from build123d import *

# Parameters (mm, degrees)
F0_R     = 11.6
F0_R_2   = 9.6
F1_DEPTH = 5.2
F2_R     = 11.6
F2_R_2   = 9.6
F3_DEPTH = 2
F4_W     = 40
F4_H     = 25
F4_R     = 11.6
F5_DEPTH = 7.2
F7_DEPTH = 1
F9_DEPTH = 1


with BuildPart() as f1:
    # F0 (on Top) → F1 (new body)
    with BuildSketch(Plane.XY):
        Circle(F0_R)
        Circle(F0_R_2, mode=Mode.SUBTRACT)
    extrude(amount=F1_DEPTH)

    # F2 (on face) → F3 (join)
    with BuildSketch(Plane.XY.offset(5.2)):
        Circle(F2_R)
        Circle(F2_R_2, mode=Mode.SUBTRACT)
        Circle(F2_R_2)
    extrude(amount=F3_DEPTH)

    # F4 (on face) → F5 (join)
    with BuildSketch(Plane.XY.offset(7.2)):
        Rectangle(F4_W, F4_H)
        Circle(F4_R, mode=Mode.SUBTRACT)
    extrude(amount=-F5_DEPTH)

    # F6 (on face) → F7 (cut)
    with BuildSketch(Plane.XY.offset(7.2)):
        Polygon((0, 2.9988845345), (-20, -12.5), (20, -12.5), align=None)
    extrude(amount=-F7_DEPTH, mode=Mode.SUBTRACT)

    # F8 (on face) → F9 (join)
    with BuildSketch(Plane.XY.offset(7.2)):
        Polygon((20, 12.5), (-20, 12.5), (-4.2277933686, -0.2774195283), (0, 2.9988845345), (4.2277933686, -0.2774195283), align=None)
        Polygon((0, 2.9988845345), (-4.2277933686, -0.2774195283), (0, -3.702450078), (4.2277933686, -0.2774195283), align=None)
    extrude(amount=F9_DEPTH)


solid = f1.part
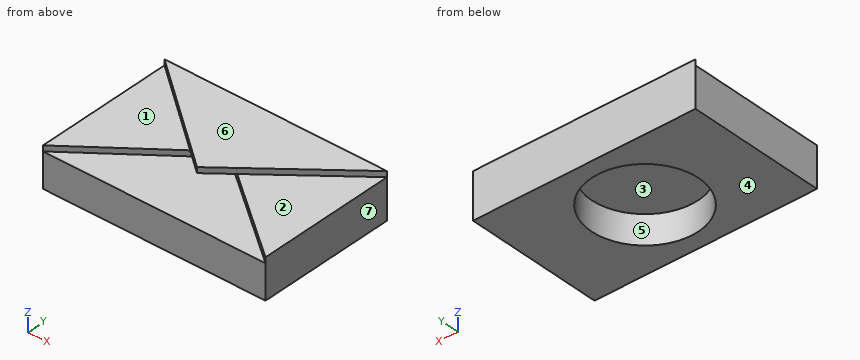
The model under review builds one solid part; all positions refer to its coordinate system, in mm. Face numbers are marked on the shaded views. A direction names the side the tool comes from. Round coordinates to 2 decimals unless told otherwise and drop trailing zeros. Loops run counter-clockwise (first coordinate to the right, second up) from the corner with the lowest first, then second, coordinate; pieces in that order, holes last. Notation, with made-up numbers: (47.5, 16.5) -> (60.5, 16.5) arc R11 ccw to (60.5, 21.5) -> close; hole circle Ø5 at (-23, 17). An arc over 180 degrees is marked (long way). Answer as CSV lines item,"result".
1) Tool access review of the marked faces 1, 2, 3 and 4: name each direction out of +Z, -Z, +X, -X, +Y, -Y from which nothing blocks a thin tool from reaching the whole face with its end or side.
Geometry results:
face 1,"+Z, -X, -Y"
face 2,"+Z, +X, -Y"
face 3,"-Z"
face 4,"-Z, +X, -X, +Y, -Y"
2) Add section B-B on z = 2.5. Write out the cut boundary in (x, y), plus the area to 3 significant figures.
Geometry results:
outline,"(-20, -12.5) -> (20, -12.5) -> (20, 12.5) -> (-20, 12.5) -> close; hole circle Ø19.2 at (0, 0)"
area,"710 mm²"
3) Add section C-C on y = 1.75. Write out the cut boundary in (x, z), plus the area to 3 significant figures.
Geometry results:
outline,"(-20, 0) -> (-9.44, 0) -> (-9.44, 5.2) -> (9.44, 5.2) -> (9.44, 0) -> (20, 0) -> (20, 7.2) -> (6.73, 7.2) -> (6.73, 8.2) -> (-6.73, 8.2) -> (-6.73, 7.2) -> (-20, 7.2) -> close; hole (-1.61, 6.2) -> (1.61, 6.2) -> (1.61, 7.2) -> (-1.61, 7.2) -> close"
area,"200 mm²"
4) For P1, Ø5.5, axis at x = -1.5, y = -1.5, coming from the -Z side; P2, Ø4.5, axis at x = 8.5, y = -1.5, coming from the +Z side, all flat-tipped, find the tip position at first contact; note any pin that passes through.
Geometry results:
P1,"stops at z = 5.2"
P2,"stops at z = 7.2"
5) Add section D-D on x = 13.5. Write out the cut boundary in (y, z), plus the area to 3 significant figures.
Geometry results:
outline,"(-12.5, 0) -> (12.5, 0) -> (12.5, 8.2) -> (7.23, 8.2) -> (7.23, 7.2) -> (-7.46, 7.2) -> (-7.46, 6.2) -> (-12.5, 6.2) -> close"
area,"180 mm²"
6) To check wall thickness, follow line 1 along Y through (x, z) = (0, 2.35); line 2 along Z through (x, y) = (-14, -4.5); line 3 along Z through (x, y) = (4, 2.25). State the ranges of each line that lie inside material, in increasing order. Write a range as from..to.
Geometry results:
line 1,"y = -12.5..-9.6, 9.6..12.5"
line 2,"z = 0..7.2"
line 3,"z = 5.2..8.2"
7) Draft analysis for pull direction X (two halves, no side actions). For the marked faces 5, 6 and 7, state which applies: pulls with the +X half, pulls with the -X half, needs draft (parallel to the pull), parting line crosses it, or undercut.
Geometry results:
face 5,"undercut"
face 6,"needs draft"
face 7,"pulls with the +X half"
8) Add section A-A on y = -3.25. Write out the cut boundary in (x, z).
Geometry results:
outline,"(-20, 0) -> (-9.03, 0) -> (-9.03, 5.2) -> (9.03, 5.2) -> (9.03, 0) -> (20, 0) -> (20, 7.2) -> (8.06, 7.2) -> (8.06, 6.2) -> (-8.06, 6.2) -> (-8.06, 7.2) -> (-20, 7.2) -> close; (-0.56, 7.2) -> (0.56, 7.2) -> (0.56, 8.2) -> (-0.56, 8.2) -> close"
